from build123d import *

# Parameters (mm, degrees)
SKETCH1_W           = 25.5
SKETCH1_H           = 50.5
SKETCH1_R           = 1.5
SKETCH1_W_2         = 15
SKETCH1_H_2         = 18.6
SKETCH1_W_3         = 14.8
SKETCH1_H_3         = 7.6
BOSS_EXTRUDE1_DEPTH = 3.5
SKETCH1_4_W         = 14.8
SKETCH1_4_H         = 7.6
BOSS_EXTRUDE2_DEPTH = 10
SKETCH1_6_W         = 15
SKETCH1_6_H         = 18.6
BOSS_EXTRUDE3_DEPTH = 15.5
CHAMFER1_SIZE       = 1


with BuildPart() as part:
    # Sketch1 → Boss-Extrude1 (new body)
    # profile 1 of 4: a face of its own
    with BuildSketch(Plane.XY):
        with Locations((12.75, 25.25)):
            Rectangle(SKETCH1_W, SKETCH1_H)
        with Locations((2.5, 2.5)):
            Circle(SKETCH1_R, mode=Mode.SUBTRACT)
        with Locations((2.5, 48)):
            Circle(SKETCH1_R, mode=Mode.SUBTRACT)
        with Locations((23, 2.5)):
            Circle(SKETCH1_R, mode=Mode.SUBTRACT)
        with Locations((23, 48)):
            Circle(SKETCH1_R, mode=Mode.SUBTRACT)
        with Locations((12.75, 28.74855078)):
            Rectangle(SKETCH1_W_2, SKETCH1_H_2, mode=Mode.SUBTRACT)
        with Locations((12.75, 44.2)):
            Rectangle(SKETCH1_W_3, SKETCH1_H_3, mode=Mode.SUBTRACT)
        with Locations((12.75, 6.3)):
            Rectangle(SKETCH1_W_3, SKETCH1_H_3, mode=Mode.SUBTRACT)
    # profile 2 of 4: a face of its own
    with BuildSketch(Plane.XY):
        with Locations((12.75, 44.2)):
            Rectangle(SKETCH1_W_3, SKETCH1_H_3)
    # profile 3 of 4: a face of its own
    with BuildSketch(Plane.XY):
        with Locations((12.75, 28.74855078)):
            Rectangle(SKETCH1_W_2, SKETCH1_H_2)
    # profile 4 of 4: a face of its own
    with BuildSketch(Plane.XY):
        with Locations((12.75, 6.3)):
            Rectangle(SKETCH1_W_3, SKETCH1_H_3)
    extrude(amount=-BOSS_EXTRUDE1_DEPTH)

    # Sketch1_4 → Boss-Extrude2 (add)
    with BuildSketch(Plane.XY):
        with Locations((12.75, 44.2)):
            Rectangle(SKETCH1_4_W, SKETCH1_4_H)
        with Locations((12.75, 6.3)):
            Rectangle(SKETCH1_4_W, SKETCH1_4_H)
    extrude(amount=BOSS_EXTRUDE2_DEPTH)

    # Sketch1_6 → Boss-Extrude3 (add)
    with BuildSketch(Plane.XY):
        with Locations((12.75, 28.74855078)):
            Rectangle(SKETCH1_6_W, SKETCH1_6_H)
    extrude(amount=BOSS_EXTRUDE3_DEPTH)

    # Chamfer1
    chamfer1_edges = [part.edges().sort_by_distance(p)[0] for p in [
        (0, 0, -1.75),
        (0, 50.5, -1.75),
        (25.5, 50.5, -1.75),
        (25.5, 0, -1.75),
    ]]
    chamfer(chamfer1_edges, length=CHAMFER1_SIZE)


solid = part.part
Design review of the part built by this model. Coordinates are the model's own, in mm. A direction names the side the tool comes from. Coordinates: 2 decimals unless noted, no trailing zeros. Write each loop counter-clockwise with the first axis right and the second up, starting at its lowest first coordinate (ties: lowest second). Pieces come first, ordered by that corner, then holes. Notation, with made-up numbers: (-17.75, 41) - (20.25, 41) arc R17 ccw to (20.25, 64) - close; hole circle Ø10 at (70, -26.75). An arc over 180 degrees is marked (long way). Use one line per item in the form item = value.
Q1. Consider section A-A (x = 23). Write out the cut boundary in (y, z).
Taken from the geometry:
outline = (0, -3.5) - (1, -3.5) - (1, 0) - (0, 0) - close; (4, -3.5) - (46.5, -3.5) - (46.5, 0) - (4, 0) - close; (49.5, -3.5) - (50.5, -3.5) - (50.5, 0) - (49.5, 0) - close
Q2. For probe 1 along Y at (x, z) = (18.5, 3); probe 2 along Y at (x, z) = (23, -2.05); probe 3 along Z at (x, y) = (4.25, 4), list the stretches that pass through material, from the lowest coordinate up.
Taken from the geometry:
probe_1 = 2.5 to 10.1, 19.45 to 38.05, 40.4 to 48
probe_2 = 0 to 1, 4 to 46.5, 49.5 to 50.5
probe_3 = -3.5 to 0
Q3. Machinability: for faces 1 (the flat face through (20.25, 29, 8)), 2 (the flat face through (5.35, 6, 5)), 3 (the flat face through (13, 2.5, 5)), which of the approach directions +Z, -Z, +X, -X, +Y, -Y give a long, thin tool a straight path to every point of the face, cutting with its end or side? Answer none if there is none.
Taken from the geometry:
face_1 = +Z, +X, +Y, -Y
face_2 = +Z, -X, -Y
face_3 = +Z, +X, -X, -Y
Q4. Insertion check: pin 1 Ø6 at (x, y) = (13.5, 43) entering from +Z; pin 2 Ø5 at (x, z) = (11, 5.5) entering from -Y; pin 3 Ø10 at (y, z) = (6, 9) entering from +X. Each pin has a flat end and moves straight along its axis. Give the tip position at first contact, or say it passes through.
Taken from the geometry:
pin_1 = 10
pin_2 = 2.5
pin_3 = 20.15
Q5. Consider section C-C (y = 25). Write out the cut boundary in (x, z), plus the area to 3 significant figures.
Taken from the geometry:
outline = (0, -3.5) - (25.5, -3.5) - (25.5, 0) - (20.25, 0) - (20.25, 15.5) - (5.25, 15.5) - (5.25, 0) - (0, 0) - close
area = 322 mm^2
Q6. The part is to be moulded in two halves that separate along Y. For faces 4 (the flat face through (13, 19.449, 8)), 5 (the flat face through (13, 0, -2)), 6 (the flat face through (5.25, 29, 8)), say which applies: +Y half, -Y half, draft (parallel to the pull), parting line (faces both ways), or undercut.
Taken from the geometry:
face_4 = undercut
face_5 = -Y half
face_6 = draft
Q7. Consider section B-B (z = 0.5). Write out the cut boundary in (x, y).
Taken from the geometry:
outline = (5.25, 19.45) - (20.25, 19.45) - (20.25, 38.05) - (5.25, 38.05) - close; (5.35, 2.5) - (20.15, 2.5) - (20.15, 10.1) - (5.35, 10.1) - close; (5.35, 40.4) - (20.15, 40.4) - (20.15, 48) - (5.35, 48) - close
Q8. Consider section D-D (x = 12). Write out the cut boundary in (y, z), plus the area to 3 significant figures.
Taken from the geometry:
outline = (0, -3.5) - (50.5, -3.5) - (50.5, 0) - (48, 0) - (48, 10) - (40.4, 10) - (40.4, 0) - (38.05, 0) - (38.05, 15.5) - (19.45, 15.5) - (19.45, 0) - (10.1, 0) - (10.1, 10) - (2.5, 10) - (2.5, 0) - (0, 0) - close
area = 617 mm^2
